```python
from build123d import *

# Parameters (mm, degrees)
SKETCH1_W           = 22.6314
SKETCH1_H           = 12.3952
BOSS_EXTRUDE1_DEPTH = 22.7584
BOSS_EXTRUDE2_DEPTH = 4.445
SKETCH3_R           = 3.46075
BOSS_EXTRUDE3_DEPTH = 4.7244
SKETCH4_R           = 0.53975
BOSS_EXTRUDE4_DEPTH = 1.524
BOSS_EXTRUDE5_DEPTH = 2.3114
SKETCH6_R           = 1.27
CUT_EXTRUDE1_DEPTH  = 4.7244


with BuildPart() as part:
    # Sketch1 → Boss-Extrude1 (new body)
    with BuildSketch(Plane(origin=(0, 0, 0), x_dir=(1, 0, 0), z_dir=(0, 1, 0))):
        Rectangle(SKETCH1_W, SKETCH1_H)
    extrude(amount=BOSS_EXTRUDE1_DEPTH)

    # Sketch2 → Boss-Extrude2 (add)
    with BuildSketch(Plane(origin=(0, 22.7584, 0), x_dir=(1, 0, 0), z_dir=(0, 1, 0))):
        with BuildLine():
            ThreePointArc((-0.330343341, -2.953762164), (11.3157, 0), (-0.330343341, 2.953762164))
            ThreePointArc((-0.330343341, 2.953762164), (-3.4671, 0), (-0.330343341, -2.953762164))
        make_face()
    extrude(amount=BOSS_EXTRUDE2_DEPTH)

    # Sketch3 → Boss-Extrude3 (add)
    with BuildSketch(Plane(origin=(0, 27.2034, 0), x_dir=(1, 0, 0), z_dir=(0, 1, 0))):
        with Locations((5.1181, 0)):
            Circle(SKETCH3_R)
    extrude(amount=BOSS_EXTRUDE3_DEPTH)

    # Sketch4 → Boss-Extrude4 (add)
    with BuildSketch(Plane(origin=(0, 31.9278, 0), x_dir=(1, 0, 0), z_dir=(0, 1, 0))):
        with BuildLine():
            Line((5.472274966, 3.44257907), (19.164005668, 2.033964148))
            ThreePointArc((19.164005668, 2.033964148), (20.99945, 0), (19.164005668, -2.033964148))
            Line((19.164005668, -2.033964148), (5.472274966, -3.44257907))
            ThreePointArc((5.472274966, -3.44257907), (1.65735, 0), (5.472274966, 3.44257907))
        make_face()
        with Locations((11.7856, 0)):
            Circle(SKETCH4_R, mode=Mode.SUBTRACT)
        with Locations((9.6901, 0)):
            Circle(SKETCH4_R, mode=Mode.SUBTRACT)
        with Locations((13.8811, 0)):
            Circle(SKETCH4_R, mode=Mode.SUBTRACT)
        with Locations((15.9766, 0)):
            Circle(SKETCH4_R, mode=Mode.SUBTRACT)
        with Locations((18.0721, 0)):
            Circle(SKETCH4_R, mode=Mode.SUBTRACT)
        with Locations((20.1676, 0)):
            Circle(SKETCH4_R, mode=Mode.SUBTRACT)
    extrude(amount=-BOSS_EXTRUDE4_DEPTH)

    # Sketch5 → Boss-Extrude5 (add)
    with BuildSketch(Plane(origin=(0, 18.3007, 0), x_dir=(1, 0, 0), z_dir=(0, 1, 0))):
        with BuildLine():
            Line((-16.1544, -6.1976), (16.1544, -6.1976))
            Line((16.1544, -6.1976), (16.1544, -0.7493))
            Line((16.1544, -0.7493), (15.029529043, -0.7493))
            ThreePointArc((15.029529043, -0.7493), (12.6492, 0), (15.029529043, 0.7493))
            Line((15.029529043, 0.7493), (16.1544, 0.7493))
            Line((16.1544, 0.7493), (16.1544, 6.1976))
            Line((16.1544, 6.1976), (-16.1544, 6.1976))
            Line((-16.1544, 6.1976), (-16.1544, 0.7493))
            Line((-16.1544, 0.7493), (-15.029529043, 0.7493))
            ThreePointArc((-15.029529043, 0.7493), (-12.6492, 0), (-15.029529043, -0.7493))
            Line((-15.029529043, -0.7493), (-16.1544, -0.7493))
            Line((-16.1544, -0.7493), (-16.1544, -6.1976))
        make_face()
    extrude(amount=-BOSS_EXTRUDE5_DEPTH)

    # Sketch6 → Cut-Extrude1 (cut)
    with BuildSketch(Plane(origin=(0, 31.9278, 0), x_dir=(1, 0, 0), z_dir=(0, 1, 0))):
        with Locations((5.1181, 0)):
            Circle(SKETCH6_R)
    extrude(amount=-CUT_EXTRUDE1_DEPTH, mode=Mode.SUBTRACT)


solid = part.part
```
Check sheet for the modelled part. Datum: model origin and axes. Units: mm. A direction names the side the tool comes from. Give positions to 0.01 mm unless a question says otherwise; leave off trailing zeros. Order: outer loops, then holes, each group sorted by start corner. A loop starts at its lowest first (then second) coordinate and runs counter-clockwise, first axis right, second up. Notation, with made-up numbers: (20, 57) -> (31, 57) arc R26 cw to (31, 71) -> close; hole circle Ø5 at (14.25, 45.5). An arc over 180 degrees is marked (long way). Return JSON: item names as keys, results as strings.
1. Cross-section at B-B, the plane x = -1.5. Record the cut outline in (y, z).
From the geometry:
{"outline": "(0, -6.2) -> (22.76, -6.2) -> (22.76, -2.79) -> (27.2, -2.79) -> (27.2, 2.79) -> (22.76, 2.79) -> (22.76, 6.2) -> (0, 6.2) -> close"}
2. Set-up check for faces 4 (the flat face through (12.41, 31.18, 2.73)), 5 (the cylindrical face through (12.3, 31.18, -0.16)), 6 (the cylindrical face through (12.65, 17.16, 0.05)), 7 (the flat face through (-16, 17, -0.749)): record each of +Z, -Z, +X, -X, +Y, -Y from which the full face is reachable in a straight line by a thin tool's end or side.
From the geometry:
{"face 4": "+Z, +X, +Y", "face 5": "+Y", "face 6": "-Y", "face 7": "-X, +Y, -Y"}
3. Material ranges on probe 1 along X at (y, z) = (28.7, 0); probe 2 along Y at (x, z) = (15.5, 1.5); probe 3 along Y at (x, z) = (8.5, 2.5), recorded low to high. Write a range as [from, to].
From the geometry:
{"probe 1": "[1.66, 3.85], [6.39, 8.58]", "probe 2": "[15.99, 18.3], [30.4, 31.93]", "probe 3": "[0, 27.2], [30.4, 31.93]"}
4. Go/stop test with flat-tipped pins: P1, Ø2, axis at y = 12.5, z = -5, coming from the -X side; P2, Ø2, axis at y = 22, z = 0, coming from the +X side; P3, Ø2.5, axis at y = 17, z = -4.5, coming from the +X side. Record where each tip stops, or that it passes through.
From the geometry:
{"P1": "x = -11.32", "P2": "x = 11.32", "P3": "x = 16.15"}
5. Cross-section at C-C, the plane y = 29.5. Record the cut outline in (x, z), plus the area to 3 significant figures.
From the geometry:
{"outline": "circle Ø6.92 at (5.12, 0); hole circle Ø2.54 at (5.12, 0)", "area": "32.6 mm^2"}
6. Cross-section at D-D, the plane z = -5. Record the cut outline in (x, y).
From the geometry:
{"outline": "(-16.15, 15.99) -> (-11.32, 15.99) -> (-11.32, 0) -> (11.32, 0) -> (11.32, 15.99) -> (16.15, 15.99) -> (16.15, 18.3) -> (11.32, 18.3) -> (11.32, 22.76) -> (8.78, 22.76) -> (8.78, 27.2) -> (1.46, 27.2) -> (1.46, 22.76) -> (-11.32, 22.76) -> (-11.32, 18.3) -> (-16.15, 18.3) -> close"}
7. Cross-section at A-A, the plane y = 16.5. Record the cut outline in (x, z), plus the area to 3 significant figures.
From the geometry:
{"outline": "(-16.15, -6.2) -> (16.15, -6.2) -> (16.15, -0.75) -> (15.03, -0.75) arc R1.31 cw (long way) to (15.03, 0.75) -> (16.15, 0.75) -> (16.15, 6.2) -> (-16.15, 6.2) -> (-16.15, 0.75) -> (-15.03, 0.75) arc R1.31 cw (long way) to (-15.03, -0.75) -> (-16.15, -0.75) -> close", "area": "387 mm^2"}
8. Mould release check, pull along X, two halves, no side actions. Record for faces 1 (the flat face through (-11.316, 8, 0)), 2 (the flat face through (0, 12, 6.198)), 3 (the cylindrical face through (-12.65, 17.16, -0.05)): +X half, -X half, draft (parallel to the pull), parting line (faces both ways), or undercut.
From the geometry:
{"face 1": "-X half", "face 2": "draft", "face 3": "undercut"}
